```python
from build123d import *

# Parameters (mm, degrees)
SKETCH1_R           = 2.5
BOSS_EXTRUDE1_DEPTH = 5
BOSS_EXTRUDE2_START = -5
SKETCH2_R           = 2.5
BOSS_EXTRUDE2_DEPTH = 5


with BuildPart() as part:
    # Sketch1 → Boss-Extrude1 (new body)
    with BuildSketch(Plane(origin=(0, 0, 0), x_dir=(1, 0, 0), z_dir=(0, 1, 0))):
        with BuildLine():
            Line((0, 5), (22.5, 5))
            ThreePointArc((22.5, 5), (27.5, 0), (22.5, -5))
            Line((22.5, -5), (0, -5))
            ThreePointArc((0, -5), (-5, 0), (0, 5))
        make_face()
        with Locations(Location((0, 0, 0), (0, 0, 270))):
            Circle(SKETCH1_R, mode=Mode.SUBTRACT)
        with Locations(Location((22.5, 0, 0), (0, 0, 270))):
            Circle(SKETCH1_R, mode=Mode.SUBTRACT)
    extrude(amount=BOSS_EXTRUDE1_DEPTH)

    # Sketch2 → Boss-Extrude2 (add)
    with BuildSketch(Plane(origin=(0, 5, 0), x_dir=(1, 0, 0), z_dir=(0, 1, 0)).offset(BOSS_EXTRUDE2_START)):
        with BuildLine():
            Line((2.5, -4.330127019), (-19.150635095, -16.830127019))
            ThreePointArc((-19.150635095, -16.830127019), (-25.980762114, -15), (-24.150635095, -8.169872981))
            Line((-24.150635095, -8.169872981), (-2.5, 4.330127019))
            ThreePointArc((-2.5, 4.330127019), (4.330127019, 2.5), (2.5, -4.330127019))
        make_face()
        with Locations(Location((-21.650635095, -12.5, 0), (0, 0, 270))):
            Circle(SKETCH2_R, mode=Mode.SUBTRACT)
        with Locations(Location((0, 0, 0), (0, 0, 270))):
            Circle(SKETCH2_R, mode=Mode.SUBTRACT)
    extrude(amount=BOSS_EXTRUDE2_DEPTH)


solid = part.part
```
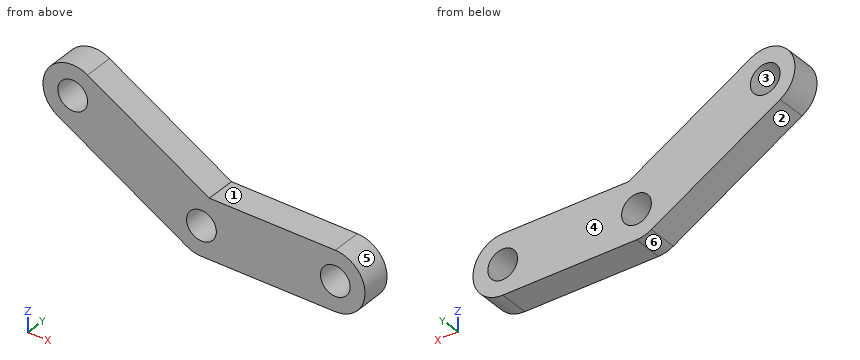
Here's how the part is built. I have some questions about the finished solid (model axes, mm). Face numbers are marked on the shaded views. A direction names the side the tool comes from. Coordinates: 2 decimals unless noted, no trailing zeros. Write each loop counter-clockwise with the first axis right and the second up, starting at its lowest first coordinate (ties: lowest second). Pieces come first, ordered by that corner, then holes. Notation, with made-up numbers: M 11,73 L 25,73 A18 cw 25,107 Z; hole C -12.5,44.5 d1. An arc over 180 degrees is marked long. Answer as CSV lines item,"result". Start each with the question number.
Q1. If we mould it in two halves opening along Z, with no side actions, what happens to the marked faces 3, 4, 5 and 6? For each: pulls with the +Z half, pulls with the -Z half, needs draft (parallel to the pull), parting line crosses it, or undercut.
Q2. Suppose I cut it at A-A, the plane z = 0. List the corners of the cut face in (x, y) for me.
Q3. Suppose I cut it at D-D, the plane x = 10.5. List the corners of the cut face in (y, z) for me, then the cut area to 3 significant figures.
Q4. I need wall thicknesses on probe 1 along X at (y, z) = (1.55, 0); probe 2 along X at (y, z) = (4.25, 1); probe 3 along X at (y, z) = (2.15, 12.25). Which ranges of each line are inside material? Lowest first, please. Write a range as [from, to].
Q5. Suppose I cut it at B-B, the plane z = 12.5. List the corners of the cut face in (x, y) for me.
Q6. Will this pin go through, and if not, where does the flat tip stop? pin 1 Ø1 at (y, z) = (2.5, 8) entering from -X.
Q7. Suppose I cut it at C-C, the plane y = 0.65. List the corners of the cut face in (x, z) for me, then the cut area to 3 significant figures.
Q8. For the marked faces 1 and 2, which set-ups out of +Z, -Z, +X, -X, +Y, -Y let a thin tool reach every point of the face, with its end or its side?
Entries:
1,face 3,"undercut"
1,face 4,"needs draft"
1,face 5,"parting line crosses it"
1,face 6,"pulls with the -Z half"
2,outline,"M -10,0 L -2.5,0 L -2.5,5 L -10,5 Z; M 2.5,0 L 20,0 L 20,5 L 2.5,5 Z; M 25,0 L 27.5,0 L 27.5,5 L 25,5 Z"
3,outline,"M 0,-5 L 5,-5 L 5,5 L 0,5 Z"
3,area,"50.0 mm²"
4,probe 1,"x = [-10, -2.5], [2.5, 20], [25, 27.5]"
4,probe 2,"x = [-11.73, -2.29], [2.29, 20.21], [24.79, 27.4]"
4,probe 3,"x = [-26.64, -24.14], [-19.16, -11.22]"
5,outline,"M -26.65,0 L -24.15,0 L -24.15,5 L -26.65,5 Z; M -19.15,0 L -11.65,0 L -11.65,5 L -19.15,5 Z"
6,pin 1,"stops at x = -24.65"
7,outline,"M -24.15,8.17 L -2.5,-4.33 A5 ccw 0,-5 L 22.5,-5 A5 ccw 22.5,5 L 1.34,5 L -19.15,16.83 A5 ccw Z; hole C -21.65,12.5 d5; hole C 0,0 d5; hole C 22.5,0 d5"
7,area,"494 mm²"
8,face 1,"+Z, +X, +Y, -Y"
8,face 2,"-Z, -X, +Y, -Y"
